The listing builds one solid part. Answer for the finished solid, in the listing's coordinates (mm). A direction names the side the tool comes from. Give positions to 0.01 mm unless a question says otherwise; leave off trailing zeros. Write each loop counter-clockwise with the first axis right and the second up, starting at its lowest first coordinate (ties: lowest second). Pieces come first, ordered by that corner, then holes. Notation, with made-up numbers: (85.25, 43.5) -> (128.25, 43.5) arc R27 ccw to (128.25, 75.5) -> close; hole circle Ø3 at (19.5, 45). An arc over 180 degrees is marked (long way). One line per question, with ' | ' between items.
from build123d import *

# Parameters (mm, degrees)
F0_R     = 1.6002
F1_DEPTH = 25.4


with BuildPart() as f1:
    # F0 (on Front) → F1 (new body)
    with BuildSketch(Plane.XZ):
        with BuildLine():
            Line((0, -14.7701), (0, 0))
            Line((0, 0), (17.5133, 0))
            Line((17.5133, 0), (17.5133, 3.43781))
            ThreePointArc((17.5133, 3.43781), (16.2598, 5), (17.5133, 6.56219))
            Line((17.5133, 6.56219), (17.5133, 10))
            Line((17.5133, 10), (-10, 10))
            Line((-10, 10), (-10, -14.7701))
            Line((-10, -14.7701), (-6.581318, -14.7701))
            ThreePointArc((-6.581318, -14.7701), (-5, -13.415), (-3.418682, -14.7701))
            Line((-3.418682, -14.7701), (0, -14.7701))
        make_face()
        with Locations((-5, -5.0076)):
            Circle(F0_R, mode=Mode.SUBTRACT)
        with Locations((-5, 5)):
            Circle(F0_R, mode=Mode.SUBTRACT)
        with Locations((6.43, 5)):
            Circle(F0_R, mode=Mode.SUBTRACT)
        with BuildLine():
            Line((17.5133, 3.43781), (17.5133, 0))
            Line((17.5133, 0), (35.0266, 0))
            Line((35.0266, 0), (35.0266, -14.7701))
            Line((35.0266, -14.7701), (38.445282, -14.7701))
            ThreePointArc((38.445282, -14.7701), (40.0266, -13.415), (41.607918, -14.7701))
            Line((41.607918, -14.7701), (45.0266, -14.7701))
            Line((45.0266, -14.7701), (45.0266, 10))
            Line((45.0266, 10), (17.5133, 10))
            Line((17.5133, 10), (17.5133, 6.56219))
            ThreePointArc((17.5133, 6.56219), (18.861462, 6.248084), (19.4602, 5))
            ThreePointArc((19.4602, 5), (18.861462, 3.751916), (17.5133, 3.43781))
        make_face()
        with Locations((40.0266, -5.0076)):
            Circle(F0_R, mode=Mode.SUBTRACT)
        with Locations((29.29, 5)):
            Circle(F0_R, mode=Mode.SUBTRACT)
        with Locations((40.0266, 5)):
            Circle(F0_R, mode=Mode.SUBTRACT)
        with BuildLine():
            Line((38.445282, -14.7701), (35.0266, -14.7701))
            Line((35.0266, -14.7701), (35.0266, -29.5402))
            Line((35.0266, -29.5402), (17.5133, -29.5402))
            Line((17.5133, -29.5402), (17.5133, -32.97801))
            ThreePointArc((17.5133, -32.97801), (18.861462, -33.292116), (19.4602, -34.5402))
            ThreePointArc((19.4602, -34.5402), (18.861462, -35.788284), (17.5133, -36.10239))
            Line((17.5133, -36.10239), (17.5133, -39.5402))
            Line((17.5133, -39.5402), (45.0266, -39.5402))
            Line((45.0266, -39.5402), (45.0266, -14.7701))
            Line((45.0266, -14.7701), (41.607918, -14.7701))
            ThreePointArc((41.607918, -14.7701), (41.622072, -14.892287), (41.6268, -15.0152))
            ThreePointArc((41.6268, -15.0152), (39.903687, -16.610672), (38.445282, -14.7701))
        make_face()
        with Locations((29.29, -34.5402)):
            Circle(F0_R, mode=Mode.SUBTRACT)
        with Locations((40.0266, -34.5402)):
            Circle(F0_R, mode=Mode.SUBTRACT)
        with Locations((40.0266, -25.0228)):
            Circle(F0_R, mode=Mode.SUBTRACT)
        with BuildLine():
            Line((0, -29.5402), (0, -14.7701))
            Line((0, -14.7701), (-3.418682, -14.7701))
            ThreePointArc((-3.418682, -14.7701), (-3.404528, -14.892287), (-3.3998, -15.0152))
            ThreePointArc((-3.3998, -15.0152), (-5.122913, -16.610672), (-6.581318, -14.7701))
            Line((-6.581318, -14.7701), (-10, -14.7701))
            Line((-10, -14.7701), (-10, -39.5402))
            Line((-10, -39.5402), (17.5133, -39.5402))
            Line((17.5133, -39.5402), (17.5133, -36.10239))
            ThreePointArc((17.5133, -36.10239), (16.2598, -34.5402), (17.5133, -32.97801))
            Line((17.5133, -32.97801), (17.5133, -29.5402))
            Line((17.5133, -29.5402), (0, -29.5402))
        make_face()
        with Locations((-5, -34.5402)):
            Circle(F0_R, mode=Mode.SUBTRACT)
        with Locations((6.43, -34.5402)):
            Circle(F0_R, mode=Mode.SUBTRACT)
        with Locations((-5, -25.0228)):
            Circle(F0_R, mode=Mode.SUBTRACT)
    extrude(amount=F1_DEPTH)


solid = f1.part
Item 1: Find section C-C (x = -5). Write down the section's boundary in (y, z) (3 decimals).
Answers below:
outline: (-25.4, -39.54) -> (0, -39.54) -> (0, -36.14) -> (-25.4, -36.14) -> close; (-25.4, -32.94) -> (0, -32.94) -> (0, -26.623) -> (-25.4, -26.623) -> close; (-25.4, -23.423) -> (0, -23.423) -> (0, -16.615) -> (-25.4, -16.615) -> close; (-25.4, -13.415) -> (0, -13.415) -> (0, -6.608) -> (-25.4, -6.608) -> close; (-25.4, -3.407) -> (0, -3.407) -> (0, 3.4) -> (-25.4, 3.4) -> close; (-25.4, 6.6) -> (0, 6.6) -> (0, 10) -> (-25.4, 10) -> close
Item 2: A flat-ended cylindrical pin translates along its axis: pin 1 (1.9 mm diameter, centred on x = 40.03, z = -25.02, fed in from -Y). Find the tip coordinate at first contact, or state that the pin passes through.
Answers below:
pin 1: through
Item 3: A tool of negligible diameter and unlimited length cuts with its end or side. For faces 5 (the face through (18, -13, -29.54)), 6 (the face through (17, -25.4, 2)), from which of +Z, -Z, +X, -X, +Y, -Y can it reach the whole face along a straight path? Write none if from no direction.
Answers below:
face 5: +Y, -Y | face 6: +Z, -Z, +X, -X, -Y
Item 4: Consider line 1 (Z direction, x = 6.43, y = -14.25); line 2 (Z direction, x = 11, y = -16.5); line 3 (X direction, y = -17, z = -36). Determine where each line is inside the solid, lowest interval first. Write a range as [from, to].
Answers below:
line 1: [-39.54, -36.14], [-32.94, -29.54], [0, 3.4], [6.6, 10] | line 2: [-39.54, -29.54], [0, 10] | line 3: [-10, -5.66], [-4.34, 5.77], [7.09, 17.2], [18.52, 28.63], [29.95, 39.37], [40.68, 45.03]
Item 5: Find section B-B (z = -9). Write down the section's boundary in (x, y), then the cut area to 3 significant figures.
Answers below:
outline: (-10, -25.4) -> (0, -25.4) -> (0, 0) -> (-10, 0) -> close; (35.03, -25.4) -> (45.03, -25.4) -> (45.03, 0) -> (35.03, 0) -> close | area: 508 mm²
Item 6: Find section A-A (x = 6.43). Write down the section's boundary in (y, z).
Answers below:
outline: (-25.4, -39.54) -> (0, -39.54) -> (0, -36.14) -> (-25.4, -36.14) -> close; (-25.4, -32.94) -> (0, -32.94) -> (0, -29.54) -> (-25.4, -29.54) -> close; (-25.4, 0) -> (0, 0) -> (0, 3.4) -> (-25.4, 3.4) -> close; (-25.4, 6.6) -> (0, 6.6) -> (0, 10) -> (-25.4, 10) -> close
Item 7: Determine the mould class of faces 1 (the face through (-10, -13, -14)), 2 (the face through (-4.26, -12.52, 3.58)), 3 (the face through (18, -13, 10)), 4 (the face through (35.027, -13, -15)) for opening direction X: pulls with the +X half, pulls with the -X half, needs draft (parallel to the pull), parting line crosses it, or undercut.
Answers below:
face 1: pulls with the -X half | face 2: undercut | face 3: needs draft | face 4: undercut
Item 8: Find section D-D (y = -16.25). Count the separate pieces of the cut face and the enclosed holes in it, then the cut area to 3 significant figures.
Answers below:
separate pieces: 1 | enclosed holes: 17 | area: 1,560 mm²
